```python
from build123d import *

# Parameters (mm, degrees)
CUT_EXTRUDE1_DEPTH      = 41.137264481
CUT_EXTRUDE1_DEPTH_BACK = 41.137264481
SKETCH2_R               = 3
SKETCH2_R_2             = 1


with BuildPart() as part:
    # Sketch1 → Revolve1 (revolve)
    with BuildSketch(Plane(origin=(0, 0, 0), x_dir=(0, 0, -1), z_dir=(1, 0, 0))):
        Polygon((0, 7), (0, -7), (-7.5, -7), (-7.5, -12), (-25, -12), (-25, -7), (-13.5, -7), (-13.5, 7), (-25, 7), (-25, 12), (-7.5, 12), (-7.5, 7), align=None)
    revolve(axis=Axis((0, 7, 0), (0, -1, 0)))

    # Sketch2 → Cut-Extrude1 (cut, two sides: drawn at the far end of the back side and taken through both)
    with BuildSketch(Plane.XZ.offset(7).offset(-CUT_EXTRUDE1_DEPTH_BACK)):
        with Locations(Location((0, 0, 0), (0, 0, 270))):
            Circle(SKETCH2_R)
        with Locations(Location((4, -4, 0), (0, 0, 270))):
            Circle(SKETCH2_R_2)
        with Locations(Location((-4, -4, 0), (0, 0, 270))):
            Circle(SKETCH2_R_2)
        with Locations(Location((-4, 4, 0), (0, 0, 270))):
            Circle(SKETCH2_R_2)
        with Locations(Location((4, 4, 0), (0, 0, 270))):
            Circle(SKETCH2_R_2)
    extrude(amount=CUT_EXTRUDE1_DEPTH + CUT_EXTRUDE1_DEPTH_BACK, mode=Mode.SUBTRACT)


solid = part.part
```
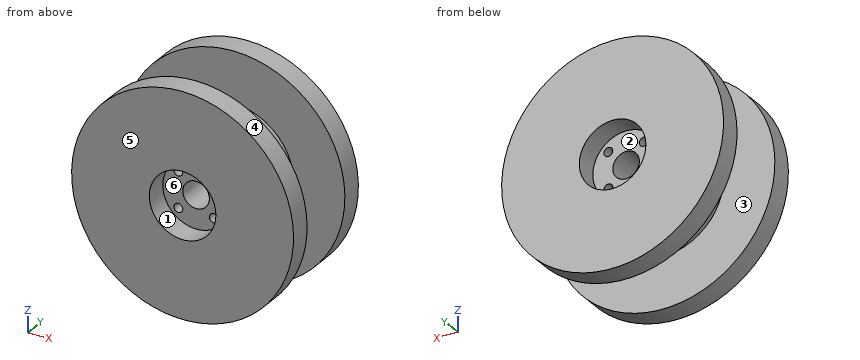
The listing builds one solid part. Answer for the finished solid, in the listing's coordinates (mm). Face numbers are marked on the shaded views. A direction names the side the tool comes from. Coordinates: 2 decimals unless noted, no trailing zeros. Write each loop counter-clockwise with the first axis right and the second up, starting at its lowest first coordinate (ties: lowest second). Pieces come first, ordered by that corner, then holes. Notation, with made-up numbers: (54, 86) - (94, 86) arc R20 ccw to (94, 106) - close; hole circle Ø6 at (48.25, 57.5). An arc over 180 degrees is marked (long way). One line per item, written item: value.
1) For a pull along Z with two mould halves and no side action, classify the marked faces 4, 5 and 6 as pulls with the +Z half, pulls with the -Z half, needs draft (parallel to the pull), parting line crosses it, or undercut.
Geometry check:
face 4: parting line crosses it
face 5: needs draft
face 6: undercut
2) Consider line 1 along Z through (x, y) = (0, 3.5); line 2 along Y through (x, z) = (-18, 17). Determine where each line is inside the solid, lowest interval first. Write a range as from..to.
Geometry check:
line 1: z = -13.5..-3, 3..13.5
line 2: y = -12..-7, 7..12
3) Find section C-C (y = -1.5). Give the vertices of the cut face in (x, z), and give its area (3 significant figures).
Geometry check:
outline: circle Ø27 at (0, 0); hole circle Ø2 at (-4, -4); hole circle Ø2 at (-4, 4); hole circle Ø6 at (0, 0); hole circle Ø2 at (4, -4); hole circle Ø2 at (4, 4)
area: 532 mm2
4) Find section D-D (y = -7.75). Give the vertices of the cut face in (x, z).
Geometry check:
outline: circle Ø50 at (0, 0); hole circle Ø15 at (0, 0)
5) Find section B-B (x = 0). Give the vertices of the cut face in (y, z), and give its area (3 significant figures).
Geometry check:
outline: (-12, -25) - (-7, -25) - (-7, -13.5) - (7, -13.5) - (7, -25) - (12, -25) - (12, -7.5) - (7, -7.5) - (7, -3) - (-7, -3) - (-7, -7.5) - (-12, -7.5) - close; (-12, 7.5) - (-7, 7.5) - (-7, 3) - (7, 3) - (7, 7.5) - (12, 7.5) - (12, 25) - (7, 25) - (7, 13.5) - (-7, 13.5) - (-7, 25) - (-12, 25) - close
area: 644 mm2
6) Each of these flat-tipped pins is pushed along its axis until it touches: pin 1 Ø15 at (x, z) = (6, -3.5) entering from +Y; pin 2 Ø12 at (y, z) = (9.5, 17) entering from +X; pin 3 Ø8 at (x, y) = (-9, -4) entering from -Z; pin 4 Ø4.5 at (x, z) = (-3, -3.5) entering from -Y. Where does it stop, or does it pass through?
Geometry check:
pin 1: stops at y = 12
pin 2: stops at x = 22.45
pin 3: stops at z = -24.18
pin 4: stops at y = -7
7) Find section A-A (z = 0). Give the vertices of the cut face in (x, y).
Geometry check:
outline: (-25, -12) - (-7.5, -12) - (-7.5, -7) - (-3, -7) - (-3, 7) - (-7.5, 7) - (-7.5, 12) - (-25, 12) - (-25, 7) - (-13.5, 7) - (-13.5, -7) - (-25, -7) - close; (3, -7) - (7.5, -7) - (7.5, -12) - (25, -12) - (25, -7) - (13.5, -7) - (13.5, 7) - (25, 7) - (25, 12) - (7.5, 12) - (7.5, 7) - (3, 7) - close
8) A tool of negligible diameter and unlimited length cuts with its end or side. For the marked faces 1, 2 and 3, from which of +Z, -Z, +X, -X, +Y, -Y can it reach the whole face along a straight path? Write none if from no direction.
Geometry check:
face 1: -Y
face 2: +Y
face 3: none
